The model under review builds one solid part; all positions refer to its coordinate system, in mm. A direction names the side the tool comes from. Give positions to 0.01 mm unless a question says otherwise; leave off trailing zeros. Loops run counter-clockwise (first coordinate to the right, second up) from the corner with the lowest first, then second, coordinate; pieces in that order, holes last. Notation, with made-up numbers: M 31,39 L 56,39 A24 ccw 56,52 Z; hole C 86.5,-28.75 d3. An arc over 180 degrees is marked long. Write item = value, one per line. Start each with the question number.
1. We need section A-A on y = 34.5. Give the boundary of the cut face in (x, z).
2. For faces 5 (the face through (17.55, 31, 35)), 6 (the face through (19, 2, 13.74)), 7 (the face through (-21.54, 4.22, 17.61)), 8 (the face through (-5.476, 1.479, 12.668)), list the 3-axis set-ups (+Z, -Z, +X, -X, +Y, -Y) from which the entire face can be reached by the end or side of a thin tool; tool diameter is ignored.
3. For pin 1 (1.5 mm diameter, centred on x = -0.5, y = 1.5, fed in from +Z); pin 2 (6 mm diameter, centred on x = 23.5, y = 14, fed in from -Z); pin 3 (2.5 mm diameter, centred on x = 1.5, y = 1, fed in from -Z); pin 4 (5.5 mm diameter, centred on x = 15, z = 133.74, fed in from +Y), all flat-tipped, find the tip position at first contact; note any pin that passes through.
4. We need section B-B on y = 47. Give the boundary of the cut face in (x, z), then the cut area to 3 significant figures.
5. Wall thickness on line 1 along Y through (x, z) = (19.5, 93); line 2 along Z through (x, y) = (-15, 15); line 3 along Z through (x, y) = (21.5, 16.5): over which ranges is each line inside the solid? List them lowest first. Write a range as from..to.
6. Draft analysis for pull direction Z (two halves, no side actions). For faces 1 (the face through (21.564, 21.937, 22.216)), 2 (the face through (26.3, 59.5, 57.4)), 3 (the face through (7.159, 44.684, 34.761)), 4 (the face through (5.476, 1.479, 12.668)), state which applies: pulls with the +Z half, pulls with the -Z half, needs draft (parallel to the pull), parting line crosses it, or undercut.
7. We need section D-D on z = 84. Give the boundary of the cut face in (x, y), then the cut area to 3 significant figures.
8. We need section C-C on y = 15.5. Give the boundary of the cut face in (x, z), then the cut area to 3 significant figures.
from build123d import *

# Parameters (mm, degrees)
SKETCH1_R           = 2
SKETCH1_W           = 30
SKETCH1_H           = 14
BOSS_EXTRUDE1_DEPTH = 3
CUT_EXTRUDE1_DEPTH  = 3
FILLET1_R           = 5
FILLET2_R           = 2
SKETCH3_W           = 45.1
SKETCH3_H           = 3
BOSS_EXTRUDE2_DEPTH = 58
FILLET3_R           = 0.5
FILLET4_R           = 1
CUT_EXTRUDE2_DEPTH  = 10
FILLET5_R           = 3
BOSS_EXTRUDE3_DEPTH = 2
FILLET6_R           = 3
SKETCH6_W           = 45.1
SKETCH6_H           = 3
BOSS_EXTRUDE4_DEPTH = 45
FILLET8_R           = 2
SKETCH7_R           = 1.7
CUT_EXTRUDE3_DEPTH  = 10
BOSS_EXTRUDE5_DEPTH = 3
SKETCH10_R          = 1.7
BOSS_EXTRUDE6_DEPTH = 3
FILLET12_R          = 5


with BuildPart() as part:
    # Sketch1 → Boss-Extrude1 (new body)
    with BuildSketch(Plane(origin=(0, 0, 0), x_dir=(1, 0, 0), z_dir=(0, 1, 0))):
        Polygon((0, 10), (-22.55, 10), (-22.55, -36.239750654), (22.55, -36.239750654), (22.55, 10), align=None)
        with Locations(Location((-17.55, -23.739750654, 0), (0, 0, 270))):
            Circle(SKETCH1_R, mode=Mode.SUBTRACT)
        with Locations((0, -23.739750654)):
            Rectangle(SKETCH1_W, SKETCH1_H, mode=Mode.SUBTRACT)
        with BuildLine():
            ThreePointArc((-3.218514532, -0.451291712), (-2.452467947, 2.132580824), (0, 3.25))
            ThreePointArc((0, 3.25), (2.132580824, 2.452467947), (3.218514532, 0.451291712))
            ThreePointArc((3.218514532, 0.451291712), (2.452467947, -2.132580824), (0, -3.25))
            ThreePointArc((0, -3.25), (-2.132580824, -2.452467947), (-3.218514532, -0.451291712))
        make_face(mode=Mode.SUBTRACT)
        with Locations(Location((17.55, -23.739750654, 0), (0, 0, 270))):
            Circle(SKETCH1_R, mode=Mode.SUBTRACT)
    extrude(amount=BOSS_EXTRUDE1_DEPTH)

    # Sketch2 → Cut-Extrude1 (cut)
    with BuildSketch(Plane(origin=(0, 3, 0), x_dir=(1, 0, 0), z_dir=(0, 1, 0))):
        with BuildLine():
            Line((-22.55, 10), (-22.55, -13.739750654))
            Line((-22.55, -13.739750654), (-12.644514973, -13.739750654))
            Line((-12.644514973, -13.739750654), (-5.905264771, -4.623618495))
            ThreePointArc((-5.905264771, -4.623618495), (-2.445456421, 7.090115859), (7.5, 0))
            ThreePointArc((7.5, 0), (7.090115859, -2.445456421), (5.905264771, -4.623618495))
            Line((5.905264771, -4.623618495), (12.644514973, -13.739750654))
            Line((12.644514973, -13.739750654), (22.55, -13.739750654))
            Line((22.55, -13.739750654), (22.55, 10))
            Line((22.55, 10), (-22.55, 10))
        make_face()
        with BuildLine():
            Line((-7.670157029, -13.739750654), (7.670157029, -13.739750654))
            Line((7.670157029, -13.739750654), (2.68876926, -7.001465551))
            ThreePointArc((2.68876926, -7.001465551), (0, -7.5), (-2.68876926, -7.001465551))
            Line((-2.68876926, -7.001465551), (-7.670157029, -13.739750654))
        make_face()
    extrude(amount=-CUT_EXTRUDE1_DEPTH, mode=Mode.SUBTRACT)

    # Fillet1
    fillet1_edges = [part.edges().sort_by_distance(p)[0] for p in [
        (5.905264771, 1.5, 4.623618495),
        (-5.905264771, 1.5, 4.623618495),
        (-12.644514973, 1.5, 13.739750654),
        (12.644514973, 1.5, 13.739750654),
    ]]
    fillet(fillet1_edges, radius=FILLET1_R)

    # Fillet2
    fillet2_edges = [part.edges().sort_by_distance(p)[0] for p in [
        (-2.68876926, 1.5, 7.001465551),
        (2.68876926, 1.5, 7.001465551),
        (7.670157029, 1.5, 13.739750654),
        (-7.670157029, 1.5, 13.739750654),
    ]]
    fillet(fillet2_edges, radius=FILLET2_R)

    # Sketch3 → Boss-Extrude2 (add)
    with BuildSketch(Plane(origin=(0, 3, 0), x_dir=(1, 0, 0), z_dir=(0, 1, 0))):
        with Locations((0, -34.739750654)):
            Rectangle(SKETCH3_W, SKETCH3_H)
    extrude(amount=BOSS_EXTRUDE2_DEPTH)

    # Fillet3
    fillet3_edges = [part.edges().sort_by_distance(p)[0] for p in [
        (15, 1.5, 16.739750654),
        (-15, 1.5, 16.739750654),
        (-15, 1.5, 30.739750654),
        (15, 1.5, 30.739750654),
    ]]
    fillet(fillet3_edges, radius=FILLET3_R)

    # Fillet4
    fillet4_edges = [part.edges().sort_by_distance(p)[0] for p in [
        (0, 3, 33.239750654),
        (0, 0, 36.239750654),
    ]]
    fillet(fillet4_edges, radius=FILLET4_R)

    # Sketch4 → Cut-Extrude2 (cut)
    with BuildSketch(Plane.XY.offset(36.239750654)):
        Polygon((-3.127501776, 31), (-17.55, 50.187359056), (-17.55, 11.812640944), align=None)
        Polygon((15.66416489, 56), (-15.66416489, 56), (0, 35.160756243), align=None)
        Polygon((17.55, 11.812640944), (17.55, 50.187359056), (3.127501776, 31), align=None)
        Polygon((15.66416489, 6), (0, 26.839243757), (-15.66416489, 6), align=None)
    extrude(amount=-CUT_EXTRUDE2_DEPTH, mode=Mode.SUBTRACT)

    # Fillet5
    fillet5_edges = [part.edges().sort_by_distance(p)[0] for p in [
        (3.127501776, 31, 34.739750654),
        (17.55, 50.187359056, 34.739750654),
        (17.55, 11.812640944, 34.739750654),
        (-15.66416489, 56, 34.739750654),
        (15.66416489, 56, 34.739750654),
        (0, 35.160756243, 34.739750654),
        (0, 26.839243757, 34.739750654),
        (15.66416489, 6, 34.739750654),
        (-15.66416489, 6, 34.739750654),
        (-17.55, 50.187359056, 34.739750654),
        (-3.127501776, 31, 34.739750654),
        (-17.55, 11.812640944, 34.739750654),
    ]]
    fillet(fillet5_edges, radius=FILLET5_R)

    # Sketch5 → Boss-Extrude3 (add)
    with BuildSketch(Plane(origin=(22.55, 0, 0), x_dir=(0, 0, -1), z_dir=(1, 0, 0))):
        Polygon((-33.239750654, 61), (-13.739750654, 3), (-15.849760206, 3), (-33.239750654, 54.724074153), align=None)
    boss_extrude3 = extrude(amount=-BOSS_EXTRUDE3_DEPTH)

    # Mirror1: Boss-Extrude3 across plane
    add(boss_extrude3.mirror(Plane.ZY))

    # Fillet6
    fillet6_edges = [part.edges().sort_by_distance(p)[0] for p in [
        (21.55, 54.724074153, 33.239750654),
        (21.55, 3, 15.849760206),
        (-21.55, 54.724074153, 33.239750654),
        (-21.55, 3, 15.849760206),
    ]]
    fillet(fillet6_edges, radius=FILLET6_R)

    # Sketch6 → Boss-Extrude4 (add)
    with BuildSketch(Plane.XY.offset(36.239750654)):
        with Locations((0, 59.5)):
            Rectangle(SKETCH6_W, SKETCH6_H)
    extrude(amount=BOSS_EXTRUDE4_DEPTH)

    # Fillet8
    fillet8_edges = [part.edges().sort_by_distance(p)[0] for p in [
        (0, 58, 36.239750654),
    ]]
    fillet(fillet8_edges, radius=FILLET8_R - 0.0001)  # a hair under: the kernel refuses the full size

    # Sketch7 → Cut-Extrude3 (cut)
    with BuildSketch(Plane.XZ.offset(-58)):
        with Locations(Location((-15, 78.739750654, 0), (0, 0, 270))):
            Circle(SKETCH7_R)
        with Locations(Location((15, 78.739750654, 0), (0, 0, 270))):
            Circle(SKETCH7_R)
    extrude(amount=-CUT_EXTRUDE3_DEPTH, mode=Mode.SUBTRACT)

    # Sketch9 → Boss-Extrude5 (add)
    with BuildSketch(Plane(origin=(0, 61, 0), x_dir=(1, 0, 0), z_dir=(0, 1, 0))):
        Polygon((-22.55, -81.239750654), (-22.55, -33.239750654), (-30, -81.239750654), align=None)
        Polygon((-22.55, -81.239750654), (-30, -81.239750654), (-30, -131.239750654), (0, -131.239750654), (0, -81.239750654), align=None)
        Polygon((22.55, -81.239750654), (0, -81.239750654), (0, -131.239750654), (30, -131.239750654), (30, -81.239750654), align=None)
        Polygon((22.55, -33.239750654), (22.55, -81.239750654), (30, -81.239750654), align=None)
    extrude(amount=-BOSS_EXTRUDE5_DEPTH)

    # Sketch10 → Boss-Extrude6 (add)
    with BuildSketch(Plane.XZ.offset(-58)):
        Polygon((-30, 136.239750654), (-30, 131.239750654), (30, 131.239750654), (30, 136.239750654), (10.586303141, 136.239750654), (7.586303141, 136.239750654), (-21.497160634, 136.239750654), (-24.497160634, 136.239750654), align=None)
        with Locations(Location((-15, 133.739750654, 0), (0, 0, 270))):
            Circle(SKETCH10_R, mode=Mode.SUBTRACT)
        with BuildLine():
            ThreePointArc((16.7, 133.739750654), (15, 132.039750654), (13.3, 133.739750654))
            ThreePointArc((13.3, 133.739750654), (15, 135.439750654), (16.7, 133.739750654))
        make_face(mode=Mode.SUBTRACT)
    extrude(amount=-BOSS_EXTRUDE6_DEPTH)

    # Fillet12
    fillet12_edges = [part.edges().sort_by_distance(p)[0] for p in [
        (-30, 59.5, 81.239750654),
        (30, 59.5, 81.239750654),
        (-30, 59.5, 136.239750654),
        (30, 59.5, 136.239750654),
    ]]
    fillet(fillet12_edges, radius=FILLET12_R)


solid = part.part
Final values:
q1.outline = M -22.55,24.33 L -20.55,24.33 L -20.55,26.44 L -22.55,26.44 Z; M -22.55,33.24 L -17.55,33.24 L -17.55,36.24 L -22.55,36.24 Z; M -5.76,33.24 L 5.76,33.24 L 5.76,36.24 L -5.76,36.24 Z; M 17.55,33.24 L 22.55,33.24 L 22.55,36.24 L 17.55,36.24 Z; M 20.55,24.33 L 22.55,24.33 L 22.55,26.44 L 20.55,26.44 Z
q2.face_5 = +Z, -Z
q2.face_6 = -Z, +X, +Y, -Y
q2.face_7 = +X, -X
q2.face_8 = +Y, -Y
q3.pin_1 = 36.24
q3.pin_2 = 16.48
q3.pin_3 = -7.5
q3.pin_4 = 61
q4.outline = M -22.55,28.53 L -20.55,28.53 L -20.55,33.24 L -8.9,33.24 L -8.9,36.24 L -22.55,36.24 Z; M 8.9,33.24 L 20.55,33.24 L 20.55,28.53 L 22.55,28.53 L 22.55,36.24 L 8.9,36.24 Z
q4.area = 101 mm²
q5.line_1 = 58..61
q5.line_2 = 33.24..36.24
q5.line_3 = 18.28..20.39, 33.24..36.24
q6.face_1 = undercut
q6.face_2 = pulls with the -Z half
q6.face_3 = needs draft
q6.face_4 = undercut
q7.outline = M -30,58 L 30,58 L 30,61 L -30,61 Z
q7.area = 180 mm²
q8.outline = M -22.55,17.94 L -20.55,17.94 L -20.55,20.05 L -22.55,20.05 Z; M -22.55,33.24 L -8.52,33.24 L -8.52,36.24 L -22.55,36.24 Z; M 8.52,33.24 L 22.55,33.24 L 22.55,36.24 L 8.52,36.24 Z; M 20.55,17.94 L 22.55,17.94 L 22.55,20.05 L 20.55,20.05 Z
q8.area = 92.6 mm²
